from build123d import *

# Parameters (mm, degrees)
SQUARE_W             = 52
SQUARE_H             = 52
CUBE_EXTRUSION_DEPTH = 52
STICK_CUT_START      = 15
STICK_HOLE_R         = 5.1
STICK_CUT_DEPTH      = 90.048032459
SKETCH12_R           = 1
CUT_EXTRUDE8_DEPTH   = 12
CUT_EXTRUDE9_START   = -12
SKETCH13_R           = 1
CUT_EXTRUDE9_DEPTH   = 12
SKETCH14_R           = 1
CUT_EXTRUDE10_DEPTH  = 12
SKETCH15_R           = 1.030667793
CUT_EXTRUDE11_DEPTH  = 12
SKETCH16_R           = 1
CUT_EXTRUDE12_DEPTH  = 12


with BuildPart() as part:
    # Square → Cube-Extrusion (new body)
    with BuildSketch(Plane.XY):
        Rectangle(SQUARE_W, SQUARE_H)
    extrude(amount=CUBE_EXTRUSION_DEPTH)

    # Stick-Hole → Stick-Cut (cut, through all)
    with BuildSketch(Plane(origin=(-28.888888889, 14.444444444, 28.888888889), x_dir=(-0.7453559924999299, -0.2981423969999719, -0.596284793999944), z_dir=(0.6666666666666667, -0.3333333333333332, -0.6666666666666667)).offset(STICK_CUT_START)):
        with Locations(Location((-14.635839315, -14.230249471, 0), (0, 0, 18.434948823))):
            Circle(STICK_HOLE_R)
    extrude(amount=-STICK_CUT_DEPTH, mode=Mode.SUBTRACT)

    # Sketch12 → Cut-Extrude8 (cut)
    with BuildSketch(Plane.XY.offset(52)):
        Circle(SKETCH12_R)
    extrude(amount=-CUT_EXTRUDE8_DEPTH, mode=Mode.SUBTRACT)

    # Sketch13 → Cut-Extrude9 (cut)
    with BuildSketch(Plane(origin=(0, 0, 0), x_dir=(-1, 0, 0), z_dir=(0, 0, -1)).offset(CUT_EXTRUDE9_START)):
        with Locations(Location((0, 0, 0), (0, 0, 180))):
            Circle(SKETCH13_R)
    extrude(amount=CUT_EXTRUDE9_DEPTH, mode=Mode.SUBTRACT)

    # Sketch14 → Cut-Extrude10 (cut)
    with BuildSketch(Plane.ZY.offset(26)):
        with Locations((10.514408983, 15.48249327)):
            Circle(SKETCH14_R)
        with Locations((20.449310987, -13.814590013)):
            Circle(SKETCH14_R)
    extrude(amount=-CUT_EXTRUDE10_DEPTH, mode=Mode.SUBTRACT)

    # Sketch15 → Cut-Extrude11 (cut)
    with BuildSketch(Plane(origin=(26, 0, 0), x_dir=(0, 0, -1), z_dir=(1, 0, 0))):
        with Locations((-33.439884797, -7.650599719)):
            Circle(SKETCH15_R)
    extrude(amount=-CUT_EXTRUDE11_DEPTH, mode=Mode.SUBTRACT)

    # Sketch16 → Cut-Extrude12 (cut)
    with BuildSketch(Plane.XZ.offset(26)):
        with Locations(Location((-9, 44.28, 0), (0, 0, 270))):
            Circle(SKETCH16_R)
    extrude(amount=-CUT_EXTRUDE12_DEPTH, mode=Mode.SUBTRACT)


solid = part.part
The listing builds one solid part. Answer for the finished solid, in the listing's coordinates (mm). A direction names the side the tool comes from. Give positions to 0.01 mm unless a question says otherwise; leave off trailing zeros. Loops run counter-clockwise (first coordinate to the right, second up) from the corner with the lowest first, then second, coordinate; pieces in that order, holes last. Notation, with made-up numbers: (-39.5, 2) - (-23.5, 2) arc R17 cw to (-23.5, 19) - close; hole circle Ø11 at (1, 55). An arc over 180 degrees is marked (long way). Use one line per item in the form item = value.
1. Find the intervals of material crossed by line 1 along X through (y, z) = (-17.75, 44.28); line 2 along Z through (x, y) = (-7, 0.5); line 3 along Y through (x, z) = (-8.5, 41), in increasing order. Write a range as [from, to].
Calculated:
line_1 = [-26, -10], [-8, 26]
line_2 = [0, 35.25], [39.81, 52]
line_3 = [-26, 0.62], [5.31, 26]
2. Section A-A on x = 0 is taken. Give the vertices of the cut face in (y, z).
Calculated:
outline = (-26, 0) - (-1, 0) - (-1, 12) - (1, 12) - (1, 0) - (26, 0) - (26, 52) - (1, 52) - (1, 40) - (-1, 40) - (-1, 52) - (-26, 52) - close
3. Given pin 1 Ø1.2 at (x, y) = (0, 0) entering from -Z; pin 2 Ø1.8 at (y, z) = (15.48, 10.51) entering from -X, each flat-ended and moving along its own axis, determine where each tip first touches the part or whether it passes through.
Calculated:
pin_1 = 12
pin_2 = -14
4. The mould has two halves that part along X. Classify faces 1 (the face through (26, 0, 26)), 2 (the face through (-14, 15, 11)), 3 (the face through (0, 0, 12)), 4 (the face through (20.084, -6.954, 34.2)): pulls with the +X half, pulls with the -X half, needs draft (parallel to the pull), parting line crosses it, or undercut.
Calculated:
face_1 = pulls with the +X half
face_2 = pulls with the -X half
face_3 = undercut
face_4 = needs draft
5. Which of the six approach directions +Z, -Z, +X, -X, +Y, -Y give full straight-line access (tool end or side, diameter ignored) to faces 5 (the face through (-9, -14, 44)), 6 (the face through (-8, 1, 34)), 7 (the face through (14, -8, 33))?
Calculated:
face_5 = -Y
face_6 = none
face_7 = +X
